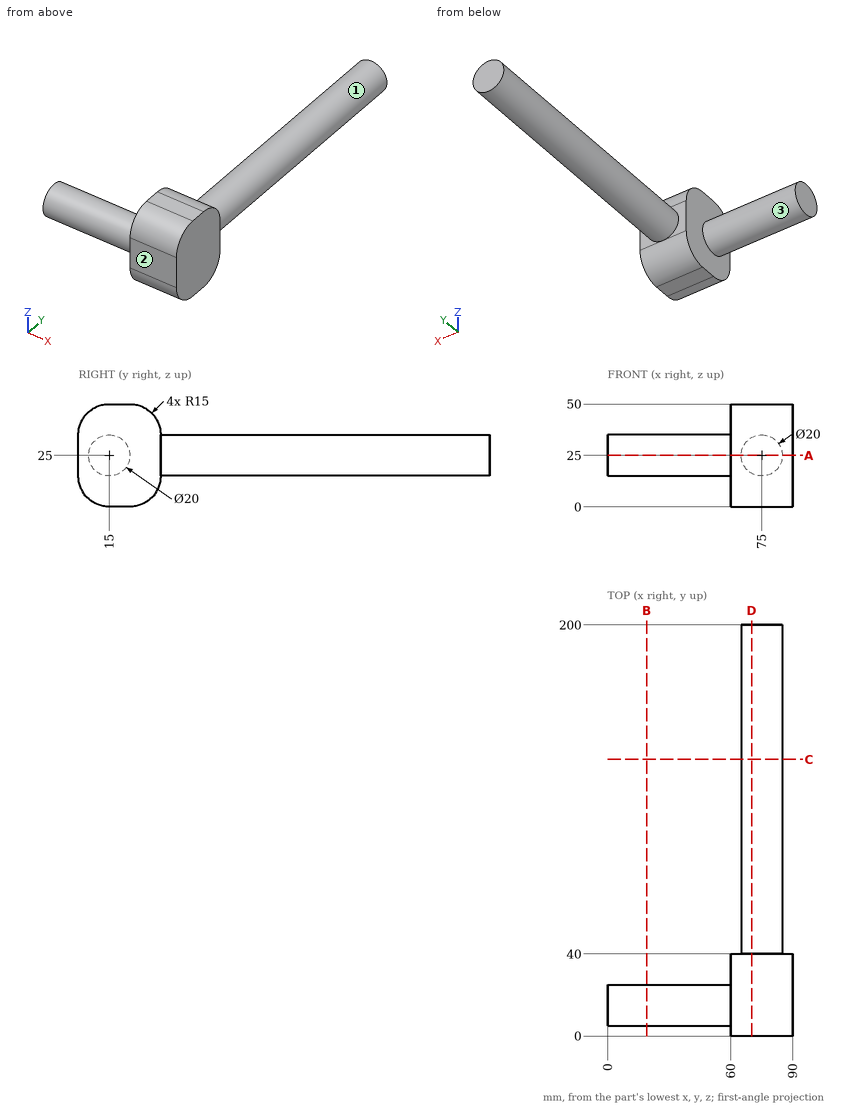
Geometry check sheet. Reference: drawing and pictorial views, mm from the part's lowest x, y, z. A direction names the side the tool comes from. Give positions to 0.01 mm unless a question says otherwise; leave off trailing zeros. Write each loop counter-clockwise with the first axis right and the second up, starting at its lowest first coordinate (ties: lowest second). Pieces come first, ordered by that corner, then holes. Notation, with made-up numbers: (62, 39.25) - (111, 39.25) arc R18 ccw to (111, 74.25) - close; hole circle Ø3 at (12.5, 6). An arc over 180 degrees is marked (long way). Use a Markdown table: item, result.
Q1. Thickness scan on L1, parallel to X at y = 22, z = 6; L2, parallel to Y at x = 84.5, z = 16.5; L3, parallel to Y at x = 81.5, z = 7. Record the ranges inside material, lowest first. Write a range as [from, to].
Computed:
| item | result |
|---|---|
| L1 | x = [60, 90] |
| L2 | y = [0, 40] |
| L3 | y = [2.31, 37.69] |
Q2. Go/stop test with flat-tipped pins: P1, Ø6, axis at x = 29.5, z = 29, coming from the -Y side; P2, Ø12, axis at y = 90.5, z = 22.5, coming from the -X side; P3, Ø5, axis at y = 95.5, z = 38, coming from the -X side; P4, Ø6, axis at x = 51, z = 13.5, coming from the +Y side. Record where each tip stops, or that it passes through.
Computed:
| item | result |
|---|---|
| P1 | stops at y = 5.05 |
| P2 | stops at x = 65 |
| P3 | passes through |
| P4 | stops at y = 20.27 |
Q3. Section check D-D, the plane x = 70. Enter the section's corners in (y, z), then the cut area to 3 significant figures.
Computed:
| item | result |
|---|---|
| outline | (0, 15) arc R15 ccw to (15, 0) - (25, 0) arc R15 ccw to (40, 15) - (40, 16.34) - (200, 16.34) - (200, 33.66) - (40, 33.66) - (40, 35) arc R15 ccw to (25, 50) - (15, 50) arc R15 ccw to (0, 35) - close |
| area | 4,580 mm² |
Q4. Set-up check for the marked faces 1, 2 and 3: record each of +Z, -Z, +X, -X, +Y, -Y from which the full face is reachable in a straight line by a thin tool's end or side.
Computed:
| item | result |
|---|---|
| face 1 | +Y |
| face 2 | +Z, -Z, +X, -X, -Y |
| face 3 | -X |
Q5. Section check C-C, the plane y = 134.5. Enter the section's corners in (x, z).
Computed:
| item | result |
|---|---|
| outline | circle Ø20 at (75, 25) |
Q6. Section check B-B, the plane x = 19. Enter the section's corners in (y, z).
Computed:
| item | result |
|---|---|
| outline | circle Ø20 at (15, 25) |
Q7. Section check A-A, the plane z = 25. Enter the section's corners in (x, y).
Computed:
| item | result |
|---|---|
| outline | (0, 5) - (60, 5) - (60, 0) - (90, 0) - (90, 40) - (85, 40) - (85, 200) - (65, 200) - (65, 40) - (60, 40) - (60, 25) - (0, 25) - close |
